The listing builds one solid part. Answer for the finished solid, in the listing's coordinates (mm). A direction names the side the tool comes from. Round coordinates to 2 decimals unless told otherwise and drop trailing zeros. Write each loop counter-clockwise with the first axis right and the second up, starting at its lowest first coordinate (ties: lowest second). Pieces come first, ordered by that corner, then holes.
(1) Each of these flat-tipped pins is pushed along its axis until it touches: pin 1 Ø3.5 at (x, y) = (140.5, 3.5) entering from +Z; pin 2 Ø3.5 at (y, z) = (5.5, 77.5) entering from +X; pin 3 Ø3.5 at (y, z) = (5, 77) entering from -X. Where does it stop, or does it pass through?
(2) For faces 1 (the face through (-3, 12, 1)), 2 (the face through (149, 6, 75)), 3 (the face through (-151, 6, 75)), 4 (the face through (-145.6, 6, 1)), determine the directions among +Z, -Z, +X, -X, +Y, -Y from which every point of the face is accessible in a straight line to the end or side of a thin tool.
(3) A cutting plane is placed at C-C, the plane x = -174. Give the vertices of the cut face in (y, z).
(4) Find the intervals of material crossed by probe 1 along X at (y, z) = (10.5, 14.5); probe 2 along Z at (x, y) = (102.5, 4.25), in increasing order.
(5) A cutting plane is placed at A-A, the plane y = 5.75. Give the vertices of the cut face in (x, z).
(6) The mould has two halves that part along Z. Classify faces 5 (the face through (200, 6, 1)), 6 (the face through (-150, 6, 1)), 7 (the face through (150, 6, 1)), 8 (the face through (-1, 6, 79.5)): +Z half, -Z half, draft (parallel to the pull), parting line (faces both ways), or undercut.
(7) A cutting plane is placed at B-B, the plane z = -12.5. Give the vertices of the cut face in (x, y), and give its area (3 significant figures).
from build123d import *

# Parameters (mm, degrees)
SKETCH1_W           = 200
SKETCH1_H           = 4.5
BOSS_EXTRUDE1_DEPTH = 12
SKETCH3_W           = 4.4
SKETCH3_H           = 75
CUT_EXTRUDE1_DEPTH  = 12


with BuildPart() as part:
    # Sketch1 → Boss-Extrude1 (new body)
    with BuildSketch(Plane(origin=(0, 0, 0), x_dir=(1, 0, 0), z_dir=(0, 1, 0))):
        Polygon((200, 75), (-200, 75), (-200, -75), (-100, -75), (-100, -70.5), (100, -70.5), (100, -75), (200, -75), align=None)
        with Locations((0, -77.25)):
            Rectangle(SKETCH1_W, SKETCH1_H)
        with Locations((0, -72.75)):
            Rectangle(SKETCH1_W, SKETCH1_H)
    extrude(amount=BOSS_EXTRUDE1_DEPTH)

    # Sketch3 → Cut-Extrude1 (cut)
    with BuildSketch(Plane(origin=(0, 12, 0), x_dir=(1, 0, 0), z_dir=(0, 1, 0))):
        with Locations((-147.8, 0)):
            Rectangle(SKETCH3_W, SKETCH3_H)
    cut_extrude1 = extrude(amount=-CUT_EXTRUDE1_DEPTH, mode=Mode.SUBTRACT)

    # Mirror1: Cut-Extrude1 across plane
    add(cut_extrude1.mirror(Plane(origin=(0, 0, 0), x_dir=(0, 0, 1), z_dir=(1, 0, 0))), mode=Mode.SUBTRACT)


solid = part.part
Solutions:
1. pin 1: stops at z = 75
1. pin 2: stops at x = 100
1. pin 3: stops at x = -100
2. face 1: +Z, -Z, +X, -X, +Y
2. face 2: +Z, +X, +Y, -Y
2. face 3: +Z, -X, +Y, -Y
2. face 4: +Y, -Y
3. outline: (0, -75) - (12, -75) - (12, 75) - (0, 75) - close
4. probe 1: x = -200 to -150, -145.6 to 145.6, 150 to 200
4. probe 2: z = -75 to 75
5. outline: (-200, -75) - (200, -75) - (200, 75) - (100, 75) - (100, 79.5) - (-100, 79.5) - (-100, 75) - (-200, 75) - close; hole (-150, -37.5) - (-145.6, -37.5) - (-145.6, 37.5) - (-150, 37.5) - close; hole (145.6, -37.5) - (150, -37.5) - (150, 37.5) - (145.6, 37.5) - close
6. face 5: draft
6. face 6: undercut
6. face 7: undercut
6. face 8: +Z half
7. outline: (-200, 0) - (-150, 0) - (-150, 12) - (-200, 12) - close; (-145.6, 0) - (145.6, 0) - (145.6, 12) - (-145.6, 12) - close; (150, 0) - (200, 0) - (200, 12) - (150, 12) - close
7. area: 4,690 mm2
